For this review, take the finished solid that the model builds, in its own axes (mm). Face numbers are marked on the shaded views. A direction names the side the tool comes from. Round coordinates to 2 decimals unless told otherwise and drop trailing zeros. Order: outer loops, then holes, each group sorted by start corner. A loop starts at its lowest first (then second) coordinate and runs counter-clockwise, first axis right, second up. Notation, with made-up numbers: (-14.5, 15.25) - (39.5, 15.25) arc R8 ccw to (39.5, 21.25) - close; hole circle Ø7 at (44, -1.75). An arc over 180 degrees is marked (long way). Write each question's results on one line, items separated by ' | '. Start each with the question number.
(1) Take a section at A-A, the plane z = 8.25. Give the boundary of the cut face in (x, y), plus the area to 3 significant figures.
(2) Take a section at D-D, the plane x = -9.75. Give the boundary of the cut face in (y, z).
(3) Take a section at C-C, the plane x = 8.5. Give the boundary of the cut face in (y, z), plus the area to 3 significant figures.
(4) For the marked faces 1 and 2, list the 3-axis set-ups (+Z, -Z, +X, -X, +Y, -Y) from which the entire face can be reached by the end or side of a thin tool; tool diameter is ignored.
(5) Insertion check: pin 1 Ø1.5 at (x, z) = (-6, 19) entering from -Y; pin 2 Ø16 at (x, y) = (0, 0) entering from +Z; pin 3 Ø1 at (x, z) = (0, 12.192) entering from -Y. Each pin has a flat end and moves straight along its axis. Give the tip position at first contact, or say it passes through.
(6) Draft analysis for pull direction Y (two halves, no side actions). For the marked faces 3, 4, 5 and 6, state which applies: pulls with the +Y half, pulls with the -Y half, needs draft (parallel to the pull), parting line crosses it, or undercut.
(7) For L1, parallel to Z at x = 0, y = 64; L2, parallel to Y at x = 0, z = 10.25; L3, parallel to Y at x = 0, z = 20.5, list the stretches that pass through material, from the lowest coordinate up. Write a range as from..to.
(8) Take a section at B-B, the plane x = 3. Give the boundary of the cut face in (y, z), plus the area to 3 significant figures.
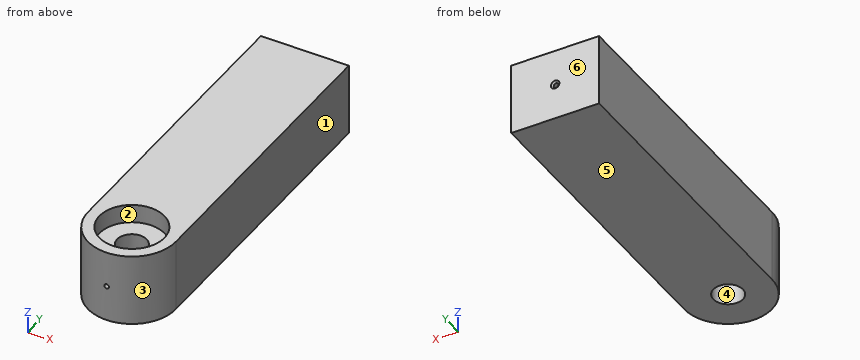
```python
from build123d import *

# Parameters (mm, degrees)
BOSS_EXTRUDE1_DEPTH                   = 24.384
F_1_16_0_0625_DOWEL_HOLE1_D           = 1.5875
F_1_16_0_0625_DOWEL_HOLE1_CSINK_D     = 2.8575
F_1_16_0_0625_DOWEL_HOLE1_CSINK_ANGLE = 100
SKETCH7_R                             = 11
CUT_EXTRUDE1_DEPTH                    = 6.25
SKETCH8_R                             = 5
CUT_EXTRUDE2_DEPTH                    = 33


with BuildPart() as part:
    # Sketch1 → Boss-Extrude1 (new body)
    with BuildSketch(Plane.XY):
        with BuildLine():
            Line((-14.859, 0), (-14.859, 101.6))
            Line((-14.859, 101.6), (14.859, 101.6))
            Line((14.859, 101.6), (14.859, 0))
            ThreePointArc((14.859, 0), (0, -14.859), (-14.859, 0))
        make_face()
    extrude(amount=BOSS_EXTRUDE1_DEPTH)

    # 1/16 (0.0625) Dowel Hole1 (through all)
    with Locations(Plane(origin=(0, 101.6, 0), x_dir=(1, 0, 0), z_dir=(0, 1, 0))):
        with Locations((0, -12.192)):
            CounterSinkHole(F_1_16_0_0625_DOWEL_HOLE1_D / 2, F_1_16_0_0625_DOWEL_HOLE1_CSINK_D / 2, counter_sink_angle=F_1_16_0_0625_DOWEL_HOLE1_CSINK_ANGLE)

    # Sketch7 → Cut-Extrude1 (cut)
    with BuildSketch(Plane.XY.offset(24.384)):
        Circle(SKETCH7_R)
    extrude(amount=-CUT_EXTRUDE1_DEPTH, mode=Mode.SUBTRACT)

    # Sketch8 → Cut-Extrude2 (cut)
    with BuildSketch(Plane.XY.offset(18.134)):
        Circle(SKETCH8_R)
    extrude(amount=-CUT_EXTRUDE2_DEPTH, mode=Mode.SUBTRACT)


solid = part.part
```
Results below:
1) outline: (-14.86, 0) arc R14.86 ccw to (14.86, 0) - (14.86, 101.6) - (-14.86, 101.6) - close; hole circle Ø10 at (0, 0) | area: 3,290 mm^2
2) outline: (-11.21, 0) - (101.6, 0) - (101.6, 24.38) - (5.09, 24.38) - (5.09, 18.13) - (-5.09, 18.13) - (-5.09, 24.38) - (-11.21, 24.38) - close
3) outline: (-12.19, 0) - (101.6, 0) - (101.6, 24.38) - (6.98, 24.38) - (6.98, 18.13) - (-6.98, 18.13) - (-6.98, 24.38) - (-12.19, 24.38) - close | area: 2,690 mm^2
4) face 1: +Z, -Z, +X, +Y, -Y | face 2: +Z
5) pin 1: stops at y = -13.9 | pin 2: stops at z = 18.13 | pin 3: passes through
6) face 3: pulls with the -Y half | face 4: undercut | face 5: needs draft | face 6: pulls with the +Y half
7) L1: z = 0..11.4, 12.99..24.38 | L2: y = -14.86..-5, 5..101.6 | L3: y = -14.86..-11, 11..101.6
8) outline: (-14.55, 0) - (-4, 0) - (-4, 18.13) - (-10.58, 18.13) - (-10.58, 24.38) - (-14.55, 24.38) - close; (4, 0) - (101.6, 0) - (101.6, 24.38) - (10.58, 24.38) - (10.58, 18.13) - (4, 18.13) - close | area: 2,550 mm^2
